Can you work these out from the drawing? Everything is in mm from the part's minimum corner. A direction names the side the tool comes from. Round coordinates to 2 decimals unless told otherwise and drop trailing zeros. Write each loop counter-clockwise with the first axis right and the second up, starting at its lowest first coordinate (ties: lowest second). Pieces come first, ordered by that corner, then holes.
Q1. For the marked faces 1, 2, 3, 4 and 5, which set-ups out of +Z, -Z, +X, -X, +Y, -Y let a thin tool reach every point of the face, with its end or its side?
Q2. Please list where these lines run through material, in increasing order: line 1 along X through (y, z) = (25.5, 7.75); line 2 along Z through (x, y) = (38, 21); line 3 along Y through (x, z) = (10.5, 6) (1 decimal).
Q3. I'm going to push flat-ended pins straight in: pin 1 Ø3 at (x, z) = (26.5, 6) entering from -Y (1 decimal); pin 2 Ø1.6 at (y, z) = (9, 5) entering from -X; pin 3 Ø4.5 at (x, z) = (23, 5.5) entering from +Y (1 decimal). Where does each tip first touch, or does it pass through?
Q4. If we section it at A-A (y = 11): Please give me the cut outline in (x, z), plus the area to 3 significant figures.
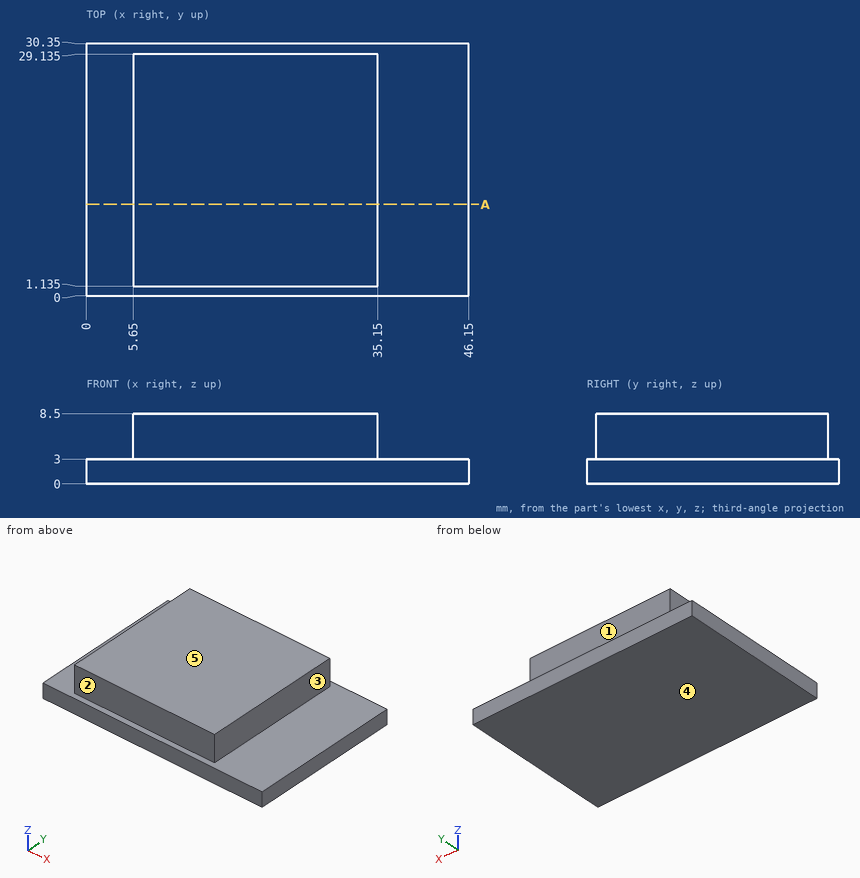
A:
1. face 1: +Z, +X, -X, +Y
1. face 2: +Z, +X, -X, -Y
1. face 3: +Z, +X, +Y, -Y
1. face 4: -Z, +X, -X, +Y, -Y
1. face 5: +Z, +X, -X, +Y, -Y
2. line 1: x = 5.65 to 35.15
2. line 2: z = 0 to 3
2. line 3: y = 1.1 to 29.1
3. pin 1: stops at y = 1.1
3. pin 2: stops at x = 5.65
3. pin 3: stops at y = 29.1
4. outline: (0, 0) - (46.15, 0) - (46.15, 3) - (35.15, 3) - (35.15, 8.5) - (5.65, 8.5) - (5.65, 3) - (0, 3) - close
4. area: 301 mm2
